Could you check a few things on this model? Use its own coordinates, in mm. Face numbers are marked on the shaded views. Coordinates: 2 decimals unless noted, no trailing zeros. Loops run counter-clockwise (first coordinate to the right, second up) from the corner with the lowest first, then second, coordinate; pieces in that order, holes last. Notation, with made-up numbers: (65, 30) -> (75, 30) arc R7 cw to (75, 35) -> close; hole circle Ø3 at (60, -13). An arc over 180 degrees is marked (long way). One line per question, with ' | ' between items. Start each with the question number.
(1) Suppose I cut it at A-A (z = 2.5). Please give me the cut outline in (x, y).
(2) I'm going to push flat-ended pins straight in: pin 1 Ø3.5 at (y, z) = (-12.5, 2.5) entering from +X; pin 2 Ø6 at (x, y) = (-5.5, 0.5) entering from -Z; pin 3 Ø2 at (y, z) = (-5, 2) entering from -X; pin 4 Ø2 at (y, z) = (1, 2.5) entering from -X. Where does each tip first touch, or does it pass through?
(3) Suppose I cut it at B-B (x = 0). Please give me the cut outline in (y, z), plus the area to 3 significant figures.
(4) If we mould it in two halves opening along Z, with no side actions, what happens to the marked faces 1, 2 and 3? For each: pulls with the +Z half, pulls with the -Z half, needs draft (parallel to the pull), parting line crosses it, or undercut.
(5) Suppose I cut it at C-C (y = 0). Please give me the cut outline in (x, z).
(6) If I drill on line 1 along Y through (x, z) = (0, 3.1); line 2 along X through (y, z) = (-10.5, 2); line 3 along Y through (x, z) = (0, 1.8), over which ranges is the centre line in solid material (lowest first)?
(7) Suppose I cut it at D-D (y = 5). Please give me the cut outline in (x, z), plus the area to 3 significant figures.
```python
from build123d import *

# Parameters (mm, degrees)
F0_R     = 10
F0_R_2   = 8.3
F1_DEPTH = 5
F2_R     = 1.5
F3_DEPTH = 2.5


with BuildPart() as f1:
    # F0 (on Top) → F1 (new body)
    with BuildSketch(Plane.XY):
        Circle(F0_R)
        Circle(F0_R_2, mode=Mode.SUBTRACT)
    extrude(amount=F1_DEPTH)

    # F2 (on Right) → F3 (join, symmetric)
    with BuildSketch(Plane.YZ):
        with BuildLine():
            Line((-9, 0), (-9, 5))
            ThreePointArc((-9, 5), (-15, 2.5), (-9, 0))
        make_face()
        with Locations((-12.5, 2.5)):
            Circle(F2_R, mode=Mode.SUBTRACT)
    extrude(amount=F3_DEPTH, both=True)


solid = f1.part
```
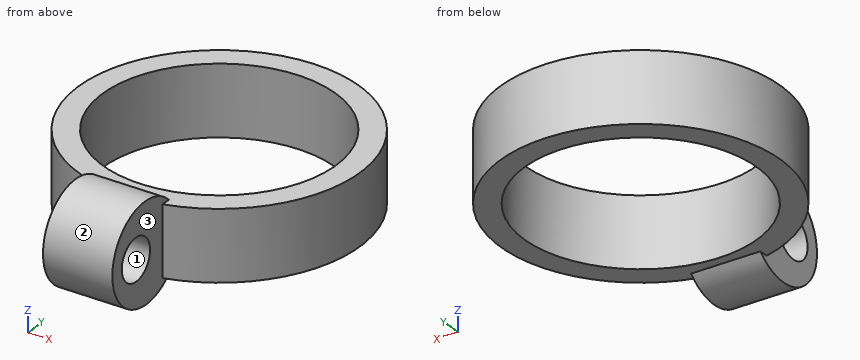
Checks:
1) outline: (-2.5, -15) -> (2.5, -15) -> (2.5, -14) -> (-2.5, -14) -> close; (-2.5, -11) -> (2.5, -11) -> (2.5, -9.68) arc R10 ccw (long way) to (-2.5, -9.68) -> close; hole circle Ø16.6 at (0, 0)
2) pin 1: stops at x = 2.5 | pin 2: stops at z = 0 | pin 3: stops at x = -9.17 | pin 4: stops at x = -10
3) outline: (-9, 0) -> (-8.3, 0) -> (-8.3, 5) -> (-9, 5) arc R3.52 ccw (long way) to start; (8.3, 0) -> (10, 0) -> (10, 5) -> (8.3, 5) -> close; hole circle Ø3 at (-12.5, 2.5) | area: 40.3 mm^2
4) face 1: undercut | face 2: parting line crosses it | face 3: needs draft
5) outline: (-10, 0) -> (-8.3, 0) -> (-8.3, 5) -> (-10, 5) -> close; (8.3, 0) -> (10, 0) -> (10, 5) -> (8.3, 5) -> close
6) line 1: y = -14.95 to -13.87, -11.13 to -8.3, 8.3 to 10 | line 2: x = -2.5 to 2.5 | line 3: y = -14.93 to -13.83, -11.17 to -8.3, 8.3 to 10
7) outline: (-8.66, 0) -> (-6.62, 0) -> (-6.62, 5) -> (-8.66, 5) -> close; (6.62, 0) -> (8.66, 0) -> (8.66, 5) -> (6.62, 5) -> close | area: 20.4 mm^2
